```python
from build123d import *

# Parameters (mm, degrees)
SKETCH1_W                      = 70
SKETCH1_H                      = 228.6
BASE_FLANGE1_DEPTH             = 0.81
EDGE_FLANGE1_STRIP_W           = 4.7132
EDGE_FLANGE1_STRIP_H           = 0.81
EDGE_FLANGE1_STRIP_CUT_DEPTH   = 228.6
EDGE_FLANGE1_DEPTH             = 228.6
EDGE_FLANGE2_STRIP_W           = 4.7132
EDGE_FLANGE2_STRIP_H           = 0.81
EDGE_FLANGE2_STRIP_CUT_DEPTH   = 228.6
EDGE_FLANGE2_DEPTH             = 228.6
EDGE_FLANGE3_STRIP_W           = 4.7132
EDGE_FLANGE3_STRIP_H           = 0.81
EDGE_FLANGE3_STRIP_CUT_DEPTH   = 68.4534
EDGE_FLANGE3_STRIP_2_W         = 4.7132
EDGE_FLANGE3_STRIP_2_H         = 0.81
EDGE_FLANGE3_STRIP_CUT_2_DEPTH = 68.4534
EDGE_FLANGE3_DEPTH             = 68.4534
EDGE_FLANGE3_BEND_DEPTH        = 68.4534
CUT_EXTRUDE2_REACH             = 255.075
SKETCH18_R                     = 2.5
SKETCH18_R_2                   = 1.5
CUT_EXTRUDE1_REACH             = 248.204
SKETCH17_R                     = 19.5
SKETCH17_R_2                   = 2.5


# Sheet-metal steps are written as plain solids
with BuildPart() as part:
    # Sketch1 → Base-Flange1 (new body)
    with BuildSketch(Plane.XY):
        with Locations((35, 114.3)):
            Rectangle(SKETCH1_W, SKETCH1_H)
    extrude(amount=-BASE_FLANGE1_DEPTH)

    # Edge-Flange1 strip (across the edge) → Edge-Flange1 strip cut (cut)
    with BuildSketch(Plane(origin=(0, 0, -0.81), x_dir=(1, 0, 0), z_dir=(0, 1, 0))):
        with Locations((-0.81, -0.405)):
            Rectangle(EDGE_FLANGE1_STRIP_W, EDGE_FLANGE1_STRIP_H)
    extrude(amount=EDGE_FLANGE1_STRIP_CUT_DEPTH, mode=Mode.SUBTRACT)

    # Edge-Flange1 section (across the edge) → Edge-Flange1 (add)
    with BuildSketch(Plane(origin=(0, 0, -0.81), x_dir=(1, 0, 0), z_dir=(0, 1, 0))):
        with BuildLine():
            Line((0, 0.7366), (0, 58))
            Line((0, 58), (0.81, 58))
            Line((0.81, 58), (0.81, 0.7366))
            ThreePointArc((0.81, 0.7366), (1.025745145, 0.215745145), (1.5466, 0))
            Line((1.5466, 0), (1.5466, -0.81))
            ThreePointArc((1.5466, -0.81), (0.452988652, -0.357011348), (0, 0.7366))
        make_face()
    extrude(amount=EDGE_FLANGE1_DEPTH)

    # Edge-Flange2 strip (across the edge) → Edge-Flange2 strip cut (cut)
    with BuildSketch(Plane(origin=(0.81, 0, -58.81), x_dir=(0, 0, 1), z_dir=(0, 1, 0))):
        with Locations((-0.81, -0.405)):
            Rectangle(EDGE_FLANGE2_STRIP_W, EDGE_FLANGE2_STRIP_H)
    extrude(amount=EDGE_FLANGE2_STRIP_CUT_DEPTH, mode=Mode.SUBTRACT)

    # Edge-Flange2 section (across the edge) → Edge-Flange2 (add)
    with BuildSketch(Plane(origin=(0.81, 0, -58.81), x_dir=(0, 0, 1), z_dir=(0, 1, 0))):
        with BuildLine():
            Line((0, 0.7366), (0, 69.19))
            Line((0, 69.19), (0.81, 69.19))
            Line((0.81, 69.19), (0.81, 0.7366))
            ThreePointArc((0.81, 0.7366), (1.025745145, 0.215745145), (1.5466, 0))
            Line((1.5466, 0), (1.5466, -0.81))
            ThreePointArc((1.5466, -0.81), (0.452988652, -0.357011348), (0, 0.7366))
        make_face()
    extrude(amount=EDGE_FLANGE2_DEPTH)

    # Edge-Flange3 strip (across the edge) → Edge-Flange3 strip cut (cut)
    with BuildSketch(Plane.YZ.offset(1.5466)):
        with Locations((-0.81, -0.405)):
            Rectangle(EDGE_FLANGE3_STRIP_W, EDGE_FLANGE3_STRIP_H)
    extrude(amount=EDGE_FLANGE3_STRIP_CUT_DEPTH, mode=Mode.SUBTRACT)

    # Edge-Flange3 strip 2 (across the edge) → Edge-Flange3 strip cut 2 (cut)
    with BuildSketch(Plane(origin=(1.5466, 0, -58), x_dir=(0, 1, 0), z_dir=(1, 0, 0))):
        with Locations((-0.81, -0.405)):
            Rectangle(EDGE_FLANGE3_STRIP_2_W, EDGE_FLANGE3_STRIP_2_H)
    extrude(amount=EDGE_FLANGE3_STRIP_CUT_2_DEPTH, mode=Mode.SUBTRACT)

    # Edge-Flange3 section (across the edge) → Edge-Flange3 (add)
    with BuildSketch(Plane.YZ.offset(1.5466)):
        with BuildLine():
            Line((0, 0.7366), (0, 24.19))
            Line((0, 24.19), (0.81, 24.19))
            Line((0.81, 24.19), (0.81, 0.7366))
            ThreePointArc((0.81, 0.7366), (1.025745145, 0.215745145), (1.5466, 0))
            Line((1.5466, 0), (1.5466, -0.81))
            ThreePointArc((1.5466, -0.81), (0.452988652, -0.357011348), (0, 0.7366))
        make_face()
    extrude(amount=EDGE_FLANGE3_DEPTH)

    # Edge-Flange3 section 2 (across the edge) → Edge-Flange3 bend (add)
    with BuildSketch(Plane(origin=(1.5466, 0, -58), x_dir=(0, 1, 0), z_dir=(1, 0, 0))):
        with BuildLine():
            Line((0, 0.7366), (0, 24.19))
            Line((0, 24.19), (0.81, 24.19))
            Line((0.81, 24.19), (0.81, 0.7366))
            ThreePointArc((0.81, 0.7366), (1.025745145, 0.215745145), (1.5466, 0))
            Line((1.5466, 0), (1.5466, -0.81))
            ThreePointArc((1.5466, -0.81), (0.452988652, -0.357011348), (0, 0.7366))
        make_face()
    extrude(amount=EDGE_FLANGE3_BEND_DEPTH)

    # Sketch18 → Cut-Extrude2 (cut, up to next)
    with BuildSketch(Plane.XY.offset(-58.81), mode=Mode.PRIVATE) as cut_extrude2_sk1:
        with Locations(Location((40, 178.288711259, 0), (0, 0, 180))):
            Circle(SKETCH18_R)
    cut_extrude2_tool1 = extrude(cut_extrude2_sk1.sketch, amount=CUT_EXTRUDE2_REACH, mode=Mode.PRIVATE) & part.part
    # Sketch18 → Cut-Extrude2 (cut, up to next)
    with BuildSketch(Plane.XY.offset(-58.81), mode=Mode.PRIVATE) as cut_extrude2_sk2:
        with Locations(Location((60, 218.6, 0), (0, 0, 180))):
            Circle(SKETCH18_R)
    cut_extrude2_tool2 = extrude(cut_extrude2_sk2.sketch, amount=CUT_EXTRUDE2_REACH, mode=Mode.PRIVATE) & part.part
    # Sketch18 → Cut-Extrude2 (cut, up to next)
    with BuildSketch(Plane.XY.offset(-58.81), mode=Mode.PRIVATE) as cut_extrude2_sk3:
        with Locations(Location((39.883110044, 168.078078525, 0), (0, 0, 180))):
            Circle(SKETCH18_R_2)
    cut_extrude2_tool3 = extrude(cut_extrude2_sk3.sketch, amount=CUT_EXTRUDE2_REACH, mode=Mode.PRIVATE) & part.part
    # Sketch18 → Cut-Extrude2 (cut, up to next)
    with BuildSketch(Plane.XY.offset(-58.81), mode=Mode.PRIVATE) as cut_extrude2_sk4:
        with Locations(Location((40, 188.499343992, 0), (0, 0, 180))):
            Circle(SKETCH18_R_2)
    cut_extrude2_tool4 = extrude(cut_extrude2_sk4.sketch, amount=CUT_EXTRUDE2_REACH, mode=Mode.PRIVATE) & part.part
    # Sketch18 → Cut-Extrude2 (cut, up to next)
    with BuildSketch(Plane.XY.offset(-58.81), mode=Mode.PRIVATE) as cut_extrude2_sk5:
        with Locations(Location((17.767718264, 178.415632815, 0), (0, 0, 180))):
            Circle(SKETCH18_R_2)
    cut_extrude2_tool5 = extrude(cut_extrude2_sk5.sketch, amount=CUT_EXTRUDE2_REACH, mode=Mode.PRIVATE) & part.part
    add(cut_extrude2_tool1.solids().sort_by_distance((40, 178.288711, -58.81))[0], mode=Mode.SUBTRACT)
    add(cut_extrude2_tool2.solids().sort_by_distance((60, 218.6, -58.81))[0], mode=Mode.SUBTRACT)
    add(cut_extrude2_tool3.solids().sort_by_distance((39.88311, 168.078079, -58.81))[0], mode=Mode.SUBTRACT)
    add(cut_extrude2_tool4.solids().sort_by_distance((40, 188.499344, -58.81))[0], mode=Mode.SUBTRACT)
    add(cut_extrude2_tool5.solids().sort_by_distance((17.767718, 178.415633, -58.81))[0], mode=Mode.SUBTRACT)

    # Sketch17 → Cut-Extrude1 (cut, up to next)
    with BuildSketch(Plane(origin=(0, 0, 0), x_dir=(-1, 0, 0), z_dir=(0, 0, -1)), mode=Mode.PRIVATE) as cut_extrude1_sk1:
        with Locations((-31.22013265, 178.33917696)):
            Circle(SKETCH17_R)
    cut_extrude1_tool1 = extrude(cut_extrude1_sk1.sketch, amount=CUT_EXTRUDE1_REACH, mode=Mode.PRIVATE) & part.part
    # Sketch17 → Cut-Extrude1 (cut, up to next)
    with BuildSketch(Plane(origin=(0, 0, 0), x_dir=(-1, 0, 0), z_dir=(0, 0, -1)), mode=Mode.PRIVATE) as cut_extrude1_sk2:
        with Locations((-60, 218.6)):
            Circle(SKETCH17_R_2)
    cut_extrude1_tool2 = extrude(cut_extrude1_sk2.sketch, amount=CUT_EXTRUDE1_REACH, mode=Mode.PRIVATE) & part.part
    add(cut_extrude1_tool1.solids().sort_by_distance((31.220133, 178.339177, 0))[0], mode=Mode.SUBTRACT)
    add(cut_extrude1_tool2.solids().sort_by_distance((60, 218.6, 0))[0], mode=Mode.SUBTRACT)


solid = part.part
```
The listing builds one solid part. Answer for the finished solid, in the listing's coordinates (mm). A direction names the side the tool comes from. Give positions to 0.01 mm unless a question says otherwise; leave off trailing zeros. Loops run counter-clockwise (first coordinate to the right, second up) from the corner with the lowest first, then second, coordinate; pieces in that order, holes last. Notation, with made-up numbers: (18, 0.5) - (28, 0.5) arc R27 ccw to (28, 25.5) - close; hole circle Ø3 at (67.25, 22.25). An arc over 180 degrees is marked (long way). Return JSON: item names as keys, results as strings. Group by question number.
1. Find section A-A (x = 65.5). Write down the section's boundary in (y, z), then the cut area to 3 significant figures.
2. Find section D-D (y = 137.5). Write down the section's boundary in (x, z).
3. Straight lines are drawn through the part: line 1 (Z direction, x = 57.5, y = 179); line 2 (Y direction, x = 40, z = -58.3); line 3 (X direction, y = 95, z = -44.5). For each, find the intervals that lie inside material, in ascending order. Write a range as [from, to].
4. Given pin 1 Ø3 at (y, z) = (154.5, -5.5) entering from +X; pin 2 Ø4 at (x, y) = (40, 188.5) entering from +Z; pin 3 Ø4 at (x, y) = (18.5, 194) entering from +Z, each flat-ended and moving along its own axis, determine where each tip first touches the part or whether it passes through.
5. Determine the mould class of faces 1 (the flat face through (35, 0.81, 13)), 2 (the flat face through (35, 117, 0)), 3 (the flat face through (35, 113, -58.81)), 4 (the flat face through (35, 0.81, -45)) for opening direction Z: pulls with the +Z half, pulls with the -Z half, needs draft (parallel to the pull), parting line crosses it, or undercut.
6. Which of the six approach directions +Z, -Z, +X, -X, +Y, -Y give full straight-line access (tool end or side, diameter ignored) to faces 5 (the cylindrical face through (35.447, 159.303, -0.399)), 6 (the flat face through (35, 117, -0.81)), 7 (the flat face through (36, 113, -58))?
7. Find section B-B (y = 218.6). Write down the section's boundary in (x, z), then the cut area to 3 significant figures.
8. Find section C-C (x = 33). Write down the section's boundary in (y, z).
Verdict:
{
 "1": {"outline": "(0, -57.26) arc R1.55 ccw to (1.55, -58.81) - (228.6, -58.81) - (228.6, -58) - (1.55, -58) arc R0.74 cw to (0.81, -57.26) - (0.81, -33.81) - (0, -33.81) - close; (0, 0.74) arc R1.55 ccw to (1.55, -0.81) - (228.6, -0.81) - (228.6, 0) - (1.55, 0) arc R0.74 cw to (0.81, 0.74) - (0.81, 24.19) - (0, 24.19) - close", "area": "409 mm^2"},
 "2": {"outline": "(0, -57.26) arc R1.55 ccw to (1.55, -58.81) - (70, -58.81) - (70, -58) - (1.55, -58) arc R0.74 cw to (0.81, -57.26) - (0.81, -1.55) arc R0.74 cw to (1.55, -0.81) - (70, -0.81) - (70, 0) - (1.55, 0) arc R1.55 ccw to (0, -1.55) - close"},
 "3": {"line 1": "z = [-58.81, -58], [-0.81, 0]", "line 2": "y = [0.4, 166.58], [169.57, 175.79], [180.79, 187], [190, 228.6]", "line 3": "x = [0, 0.81]"},
 "4": {"pin 1": "stops at x = 0.81", "pin 2": "stops at z = -58", "pin 3": "stops at z = 0"},
 "5": {"face 1": "needs draft", "face 2": "pulls with the +Z half", "face 3": "pulls with the -Z half", "face 4": "undercut"},
 "6": {"face 5": "+Z", "face 6": "+X, +Y, -Y", "face 7": "+X, +Y"},
 "7": {"outline": "(0, -57.26) arc R1.55 ccw to (1.55, -58.81) - (57.5, -58.81) - (57.5, -58) - (1.55, -58) arc R0.74 cw to (0.81, -57.26) - (0.81, -1.55) arc R0.74 cw to (1.55, -0.81) - (57.5, -0.81) - (57.5, 0) - (1.55, 0) arc R1.55 ccw to (0, -1.55) - close; (62.5, -58.81) - (70, -58.81) - (70, -58) - (62.5, -58) - close; (62.5, -0.81) - (70, -0.81) - (70, 0) - (62.5, 0) - close", "area": "151 mm^2"},
 "8": {"outline": "(0, -57.26) arc R1.55 ccw to (1.55, -58.81) - (228.6, -58.81) - (228.6, -58) - (1.55, -58) arc R0.74 cw to (0.81, -57.26) - (0.81, -33.81) - (0, -33.81) - close; (0, 0.74) arc R1.55 ccw to (1.55, -0.81) - (158.92, -0.81) - (158.92, 0) - (1.55, 0) arc R0.74 cw to (0.81, 0.74) - (0.81, 24.19) - (0, 24.19) - close; (197.76, -0.81) - (228.6, -0.81) - (228.6, 0) - (197.76, 0) - close"}
}
